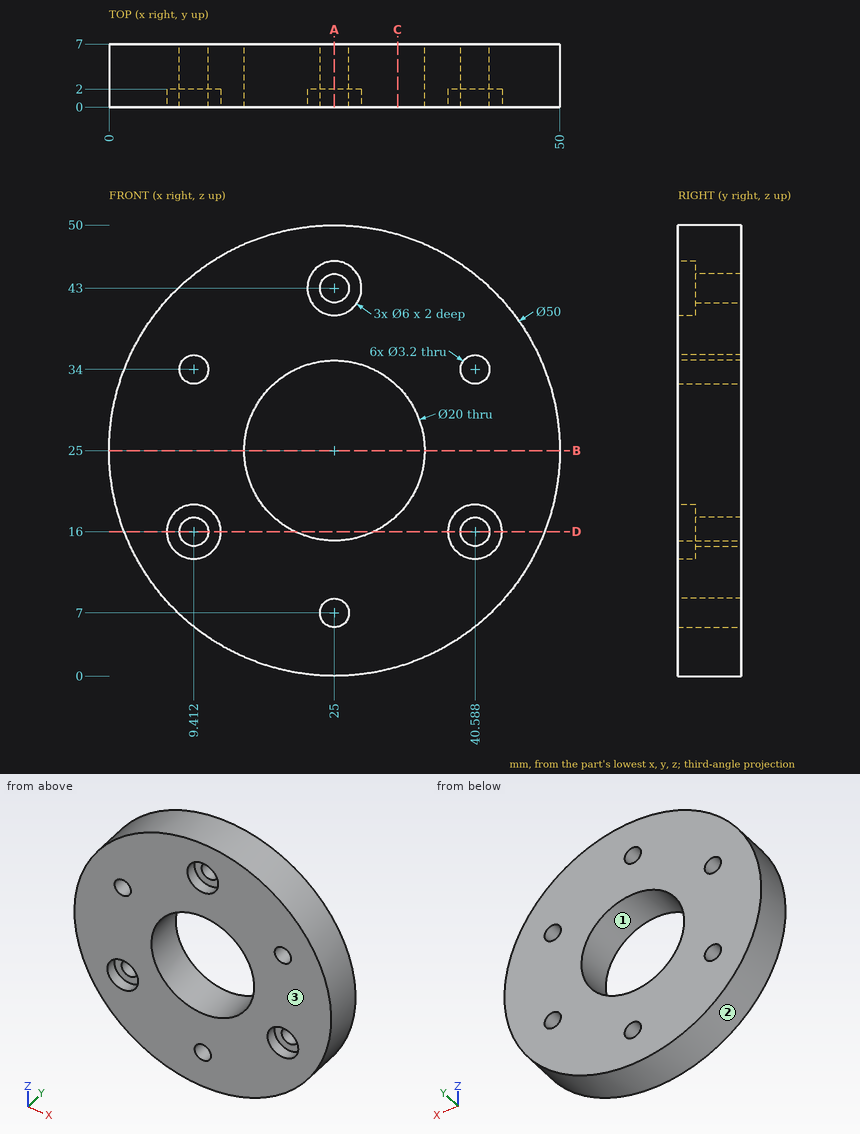
Here's the drawing with two shaded views (mm, measured from the low corner). I have some questions. Round coordinates to 2 decimals unless told otherwise and drop trailing zeros. Loops run counter-clockwise (first coordinate to the right, second up) from the corner with the lowest first, then second, coordinate; pieces in that order, holes last.
1. Suppose I cut it at A-A, the plane x = 25. Please give me the cut outline in (y, z), and give its area (3 significant figures).
Answers:
outline: (0, 0) - (7, 0) - (7, 5.4) - (0, 5.4) - close; (0, 8.6) - (7, 8.6) - (7, 15) - (0, 15) - close; (0, 35) - (7, 35) - (7, 41.4) - (2, 41.4) - (2, 40) - (0, 40) - close; (0, 46) - (2, 46) - (2, 44.6) - (7, 44.6) - (7, 50) - (0, 50) - close
area: 160 mm2
2. If I drill on probe 1 along X at (y, z) = (4, 34) (1 decimal); probe 2 along X at (y, z) = (1.35, 16) (1 decimal); probe 3 along Z at (x, y) = (27.5, 1.5) (1 decimal), over which ranges is the centre line in solid material (lowest first)?
Answers:
probe 1: x = 1.7 to 7.8, 11 to 20.6, 29.4 to 39, 42.2 to 48.3
probe 2: x = 1.7 to 6.4, 12.4 to 20.6, 29.4 to 37.6, 43.6 to 48.3
probe 3: z = 0.1 to 15.3, 34.7 to 41.3, 44.7 to 49.9
3. Suppose I cut it at C-C, the plane x = 32. Please give me the cut outline in (y, z).
Answers:
outline: (0, 1) - (7, 1) - (7, 17.86) - (0, 17.86) - close; (0, 32.14) - (7, 32.14) - (7, 49) - (0, 49) - close
4. Suppose I cut it at B-B, the plane z = 25. Please give me the cut outline in (x, y).
Answers:
outline: (0, 0) - (15, 0) - (15, 7) - (0, 7) - close; (35, 0) - (50, 0) - (50, 7) - (35, 7) - close
5. Thinking about a two-plate mould opening in Z: for the marked faces 1, 2 and 3, which applies, released by +Z, released by -Z, zero draft, split by the parting line, or undercut?
Answers:
face 1: undercut
face 2: split by the parting line
face 3: zero draft
6. Will these pins go through, and if not, where does the flat tip stop? pin 1 (4 mm diameter, centred on x = 9.41, z = 16, fed in from -Y); pin 2 (3 mm diameter, centred on x = 25, z = 7, fed in from +Y).
Answers:
pin 1: stops at y = 2
pin 2: passes through
7. Suppose I cut it at D-D, the plane z = 16. Please give me the cut outline in (x, y).
Answers:
outline: (1.68, 0) - (6.41, 0) - (6.41, 2) - (7.81, 2) - (7.81, 7) - (1.68, 7) - close; (11.01, 2) - (12.41, 2) - (12.41, 0) - (20.64, 0) - (20.64, 7) - (11.01, 7) - close; (29.36, 0) - (37.59, 0) - (37.59, 2) - (38.99, 2) - (38.99, 7) - (29.36, 7) - close; (42.19, 2) - (43.59, 2) - (43.59, 0) - (48.32, 0) - (48.32, 7) - (42.19, 7) - close
